Part model, mm, in its own coordinate system. A direction names the side the tool comes from. Give positions to 0.01 mm unless a question says otherwise; leave off trailing zeros. Write each loop counter-clockwise with the first axis right and the second up, starting at its lowest first coordinate (ties: lowest second). Pieces come first, ordered by that corner, then holes. Notation, with made-up numbers: M 38,45.25 L 79,45.25 A29 cw 79,72.25 Z; hole C 67,29.5 d7. An arc over 180 degrees is marked long. Use CSV: the item, a comma, the result in double quotes. Start each with the question number.
1. 3-axis set-ups, long thin cutter, end or side, ignore diameter. For faces 4 (the face through (-16.855, 33.986, 2.213)), 5 (the face through (0, 26.8, 0)), 6 (the face through (9.489, 3.875, 12.375)): which of +Z, -Z, +X, -X, +Y, -Y reach the whole face in a straight line?
2. Band-saw the part on C-C, the plane y = 32. List the corners of the cut face in (x, z) (3 decimals).
3. Mould opens along Z. For faces 1 (the face through (4, 35, 0)), 2 (the face through (-15.368, 17.311, 2.018)), 3 (the face through (0.07, 30.96, 2.15)) say: pulls with the +Z half, pulls with the -Z half, needs draft (parallel to the pull), parting line crosses it, or undercut.
4. Band-saw the part on A-A, the plane x = 0. List the corners of the cut face in (y, z), then the cut area to 3 significant figures.
5. Drop flat-ended pins along their axis: pin 1 Ø5 at (y, z) = (11.5, 3.5) entering from +X; pin 2 Ø1.9 at (x, z) = (1, 0.5) entering from +Y; pin 3 Ø8 at (x, y) = (-4, 17) entering from -Z. Give the stop position or say it passes through.
6. Band-saw the part on B-B, the plane z = 0. List the corners of the cut face in (x, y).
7. Drill centre lines: line 1 along X through (y, z) = (31, 0); line 2 along X through (y, z) = (33, 0); line 3 along Y through (x, z) = (9, 14). Where is each one in solid material? Low to high. Write a range as from..to.
from build123d import *

# Parameters (mm, degrees)
CUT_EXTRUDE1_DEPTH = 8.2


with BuildPart() as part:
    # Sketch1 → Revolve1 (revolve)
    with BuildSketch(Plane.XY, mode=Mode.PRIVATE) as revolve1_sk:
        Polygon((0, 0), (0, 35), (-17, 35), (-17, 33), (-15.5, 31), (-15.5, 4), (-17, 2), (-17, 0), align=None)
    revolve(revolve1_sk.sketch.rotate(Axis((0, 0, 0), (0, 1, 0)), 270), axis=Axis((0, 0, 0), (0, 1, 0)))

    # Sketch2 → Cut-Extrude1 (cut)
    with BuildSketch(Plane(origin=(0, 35, 0), x_dir=(1, 0, 0), z_dir=(0, 1, 0))):
        with BuildLine():
            Line((-1.325, 1.693184869), (1.325, 1.693184869))
            ThreePointArc((1.325, 1.693184869), (0, -2.15), (-1.325, 1.693184869))
        make_face()
    extrude(amount=-CUT_EXTRUDE1_DEPTH, mode=Mode.SUBTRACT)


solid = part.part
Output:
1,face 4,"+Y, -Y"
1,face 5,"+Y"
1,face 6,"none"
2,outline,"C 0,0 d32.5; hole M -1.325,-1.693 L 1.325,-1.693 A2.15 ccw long Z"
3,face 1,"needs draft"
3,face 2,"parting line crosses it"
3,face 3,"undercut"
4,outline,"M 0,-17 L 2,-17 L 4,-15.5 L 31,-15.5 L 33,-17 L 35,-17 L 35,-1.69 L 26.8,-1.69 L 26.8,2.15 L 35,2.15 L 35,17 L 33,17 L 31,15.5 L 4,15.5 L 2,17 L 0,17 Z"
4,area,"1,070 mm²"
5,pin 1,"stops at x = 15.47"
5,pin 2,"stops at y = 26.8"
5,pin 3,"stops at z = -15.5"
6,outline,"M -17,0 L 17,0 L 17,2 L 15.5,4 L 15.5,31 L 17,33 L 17,35 L 2.15,35 L 2.15,26.8 L -2.15,26.8 L -2.15,35 L -17,35 L -17,33 L -15.5,31 L -15.5,4 L -17,2 Z"
7,line 1,"x = -15.5..-2.15, 2.15..15.5"
7,line 2,"x = -17..-2.15, 2.15..17"
7,line 3,"y = 0..2.48, 32.52..35"
